Can you work these out from the model? Positions are in its coordinate system, mm. Face numbers are marked on the shaded views. Give positions to 0.01 mm unless a question says otherwise; leave off trailing zeros. Write each loop counter-clockwise with the first axis right and the second up, starting at its lowest first coordinate (ties: lowest second). Pieces come first, ordered by that corner, then holes. Notation, with made-up numbers: (-30.75, 46.5) - (24.25, 46.5) arc R31 cw to (24.25, 75.5) - close; hole circle Ø4 at (2, 16). An arc over 180 degrees is marked (long way). Return JSON: item names as keys, results as strings. Group by question number.
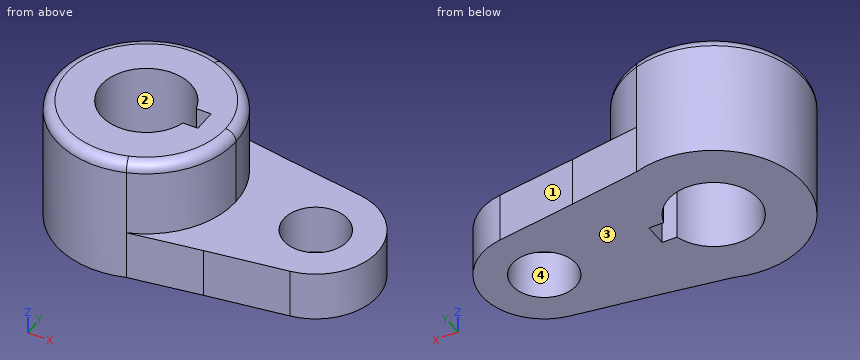
from build123d import *

# Parameters (mm, degrees)
F1_DEPTH = 40.2336
F0_R     = 10.16
F2_DEPTH = 15.7734
F3_R     = 3.302


with BuildPart() as f1:
    # F0 (on Top) → F1 (new body)
    with BuildSketch(Plane.XY):
        with BuildLine():
            ThreePointArc((9.135252, -27.075409), (23.211748, -16.665695), (28.575, 0))
            ThreePointArc((28.575, 0), (23.211748, 16.665695), (9.135252, 27.075409))
            ThreePointArc((9.135252, 27.075409), (-28.575, 0), (9.135252, -27.075409))
        make_face()
        with BuildLine():
            ThreePointArc((13.801996, -3.692906), (-14.2875, 0), (13.801996, 3.692906))
            Line((13.801996, 3.692906), (18.5293, 3.692906))
            Line((18.5293, 3.692906), (18.5293, -3.692906))
            Line((18.5293, -3.692906), (13.801996, -3.692906))
        make_face(mode=Mode.SUBTRACT)
    extrude(amount=F1_DEPTH)

    # F0 (on Top) → F2 (join)
    with BuildSketch(Plane.XY):
        with BuildLine():
            ThreePointArc((9.135252, 27.075409), (23.211748, 16.665695), (28.575, 0))
            ThreePointArc((28.575, 0), (23.211748, -16.665695), (9.135252, -27.075409))
            Line((9.135252, -27.075409), (31.555126, -23.395091))
            Line((31.555126, -23.395091), (56.972144, -19.485621))
            ThreePointArc((56.972144, -19.485621), (73.689773, 0), (56.972144, 19.485621))
            Line((56.972144, 19.485621), (31.555126, 23.395091))
            Line((31.555126, 23.395091), (9.135252, 27.075409))
        make_face()
        with Locations((53.975, 0)):
            Circle(F0_R, mode=Mode.SUBTRACT)
    extrude(amount=F2_DEPTH)

    # F3
    f3_edges = [f1.edges().sort_by_distance(p)[0] for p in [
        (-9.135252, 27.075409, 40.2336),
    ]]
    fillet(f3_edges, radius=F3_R)


solid = f1.part
1) Imagine slicing it at A-A, the plane z = 11. Count the separate pieces of the cut face and the enclosed holes in it, and give its area (3 significant figures).
2) Imagine slicing it at D-D, the plane z = 38. Write out the boundary of the cut face in (x, y) (1 decimal).
3) I need wall thicknesses on line 1 along Y through (x, z) = (0, 13.5) (1 decimal); line 2 along Z through (x, y) = (65, 3); line 3 along Y through (x, z) = (46.5, 8). Which ranges of each line are inside material? Lowest first, please.
4) We'd pull the mould along X, two halves only. Please class the marked faces 1, 2, 3 and 4: pulls with the +X half, pulls with the -X half, needs draft (parallel to the pull), parting line crosses it, or undercut.
5) Will these pins go through, and if not, where does the flat tip stop? pin 1 Ø1.5 at (y, z) = (-17.5, 8) entering from -X; pin 2 Ø4 at (x, z) = (16, 28.5) entering from -Y; pin 3 Ø2 at (y, z) = (-22.5, 8) entering from -X; pin 4 Ø12 at (x, y) = (44, -20) entering from -Z.
Resolved:
{
 "1": {"separate pieces": "1", "enclosed holes": "2", "area": "3,510 mm^2"},
 "2": {"outline": "(9.1, -26.9) arc R28.4 ccw to (28.4, 0) arc R28.4 ccw to (9.1, 26.9) arc R28.4 ccw (long way) to start; hole (13.8, -3.7) - (18.5, -3.7) - (18.5, 3.7) - (13.8, 3.7) arc R14.3 ccw (long way) to start"},
 "3": {"line 1": "-28.6 to -14.3, 14.3 to 28.6", "line 2": "0 to 15.77", "line 3": "-21.1 to -6.88, 6.88 to 21.1"},
 "4": {"face 1": "pulls with the +X half", "face 2": "undercut", "face 3": "needs draft", "face 4": "undercut"},
 "5": {"pin 1": "x = -23.15", "pin 2": "y = -24.91", "pin 3": "x = -18.82", "pin 4": "z = 0"}
}
